Read the model definition and answer for the solid it produces. Units are mm, in the model's axes. Face numbers are marked on the shaded views. A direction names the side the tool comes from. Coordinates: 2 decimals unless noted, no trailing zeros. Order: outer loops, then holes, each group sorted by start corner. A loop starts at its lowest first (then second) coordinate and runs counter-clockwise, first axis right, second up. Notation, with made-up numbers: M 63,-39 L 75,-39 A32 ccw 75,-1 Z; hole C 43.5,3.5 d7. An arc over 180 degrees is marked long. Write each question's results on one line, items separated by ' | '.
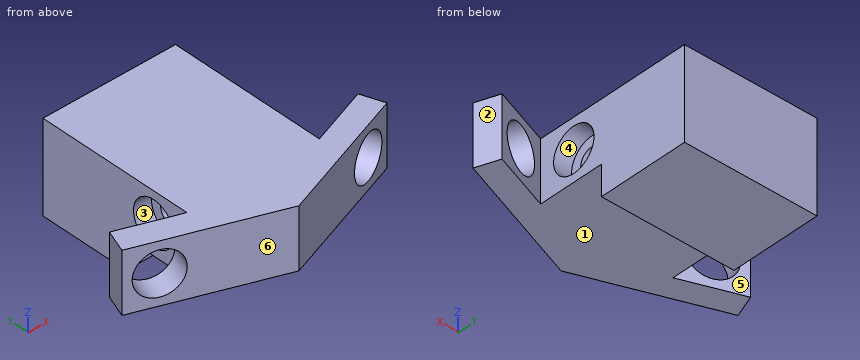
```python
from build123d import *

# Parameters (mm, degrees)
BOSS_EXTRUDE1_DEPTH = 10
SKETCH2_R           = 3.65
CUT_EXTRUDE1_DEPTH  = 16.423609234
BOSS_EXTRUDE3_DEPTH = 10
SKETCH6_R           = 3.65
CUT_EXTRUDE4_DEPTH  = 3
SKETCH8_R           = 2
CUT_EXTRUDE5_DEPTH  = 16.041318231
SKETCH9_W           = 15
SKETCH9_H           = 15
BOSS_EXTRUDE4_DEPTH = 22.041318231


with BuildPart() as part:
    # Sketch1 → Boss-Extrude1 (new body)
    with BuildSketch(Plane.XY):
        Polygon((0, 0), (20.673237657, 7.524443153), (22.041318231, 3.76567267), (0, -4.25671109), (-22.041318231, 3.76567267), (-20.673237657, 7.524443153), align=None)
    extrude(amount=BOSS_EXTRUDE1_DEPTH)

    # Sketch2 → Cut-Extrude1 (cut)
    with BuildSketch(Plane(origin=(0, 0, 0), x_dir=(0.9396926207859093, 0.34202014332566627, 0), z_dir=(-0.34202014332566627, 0.9396926207859093, 0))):
        with Locations(Location((17, -5, 0), (0, 0, 180))):
            Circle(SKETCH2_R)
    cut_extrude1 = extrude(amount=-CUT_EXTRUDE1_DEPTH, mode=Mode.SUBTRACT)

    # Mirror1: Cut-Extrude1 across plane
    add(cut_extrude1.mirror(Plane(origin=(0, 0, 0), x_dir=(0, 0, 1), z_dir=(1, 0, 0))), mode=Mode.SUBTRACT)

    # Sketch3 → Boss-Extrude3 (add)
    with BuildSketch(Plane.XY.offset(10)):
        Polygon((0, -4.25671109), (-11.020659115, -0.24551921), (-11.020659115, 15), (11.020659115, 15), (11.020659115, -0.24551921), align=None)
    extrude(amount=-BOSS_EXTRUDE3_DEPTH)

    # Sketch6 → Cut-Extrude4 (cut)
    with BuildSketch(Plane(origin=(11.020659115, 0, 0), x_dir=(0, 0, -1), z_dir=(1, 0, 0))):
        with Locations(Location((-5, 10, 0), (0, 0, 90))):
            Circle(SKETCH6_R)
    cut_extrude4 = extrude(amount=-CUT_EXTRUDE4_DEPTH, mode=Mode.SUBTRACT)

    # Mirror3: Cut-Extrude4 across plane
    add(cut_extrude4.mirror(Plane(origin=(0, 0, 0), x_dir=(0, 0, 1), z_dir=(1, 0, 0))), mode=Mode.SUBTRACT)

    # Sketch8 → Cut-Extrude5 (cut)
    with BuildSketch(Plane.ZY.offset(8.020659115)):
        with Locations(Location((5, 10, 0), (0, 0, 270))):
            Circle(SKETCH8_R)
    extrude(amount=-CUT_EXTRUDE5_DEPTH, mode=Mode.SUBTRACT)

    # Sketch9 → Boss-Extrude4 (add)
    with BuildSketch(Plane.ZY.offset(11.020659115)):
        with Locations((2.5, 22.5)):
            Rectangle(SKETCH9_W, SKETCH9_H)
    extrude(amount=-BOSS_EXTRUDE4_DEPTH)


solid = part.part
```
(1) Given pin 1 (12 mm diameter, centred on x = 5, y = 2, fed in from -Z); pin 2 (4.5 mm diameter, centred on y = 16.5, z = 3, fed in from +X); pin 3 (4.5 mm diameter, centred on y = 10, z = 5, fed in from +X), each flat-ended and moving along its own axis, determine where each tip first touches the part or whether it passes through.
Conclusion:
pin 1: z = 0 | pin 2: x = 11.02 | pin 3: x = 8.02
(2) The part is cut by section B-B, the plane z = 4.5. Count the separate pieces of the cut face and the enclosed holes in it, then the cut area to 3 significant figures.
Conclusion:
separate pieces: 4 | enclosed holes: 0 | area: 635 mm²
(3) The mould has two halves that part along Z. Classify the marked faces 1, 2 and 3: pulls with the +Z half, pulls with the -Z half, needs draft (parallel to the pull), parting line crosses it, or undercut.
Conclusion:
face 1: pulls with the -Z half | face 2: needs draft | face 3: undercut
(4) The part is cut by section A-A, the plane y = 10. Write down the section's boundary in (x, z).
Conclusion:
outline: M -11.02,0 L 11.02,0 L 11.02,1.35 L 8.02,1.35 L 8.02,3 L -8.02,3 L -8.02,1.35 L -11.02,1.35 Z; M -11.02,8.65 L -8.02,8.65 L -8.02,7 L 8.02,7 L 8.02,8.65 L 11.02,8.65 L 11.02,10 L -11.02,10 Z
(5) The part is cut by section D-D, the plane y = 24.5. Write down the section's boundary in (x, z), then the cut area to 3 significant figures.
Conclusion:
outline: M -11.02,-5 L 11.02,-5 L 11.02,10 L -11.02,10 Z | area: 331 mm²
(6) Straight lines are drawn through the part: line 1 (Z direction, x = -9, y = 10); line 2 (X direction, y = 6.5, z = 8); line 3 (X direction, y = 6, z = 3.75). For each, find the intervals that lie inside material, in ascending order.
Conclusion:
line 1: 0 to 1.35, 8.65 to 10 | line 2: -21.05 to -17.94, -11.02 to 11.02, 17.94 to 21.05 | line 3: -21.23 to -19.56, -11.02 to 11.02, 19.56 to 21.23
(7) For the marked faces 4, 5 and 6, determine the directions among +Z, -Z, +X, -X, +Y, -Y from which every point of the face is accessible in a straight line to the end or side of a thin tool.
Conclusion:
face 4: none | face 5: +Z, -Z, +Y | face 6: +Z, -Z, -X, -Y
(8) The part is cut by section C-C, the plane x = -1.5. Write down the section's boundary in (y, z).
Conclusion:
outline: M -3.71,0 L 15,0 L 15,-5 L 30,-5 L 30,10 L -3.71,10 Z; hole C 10,5 d4
